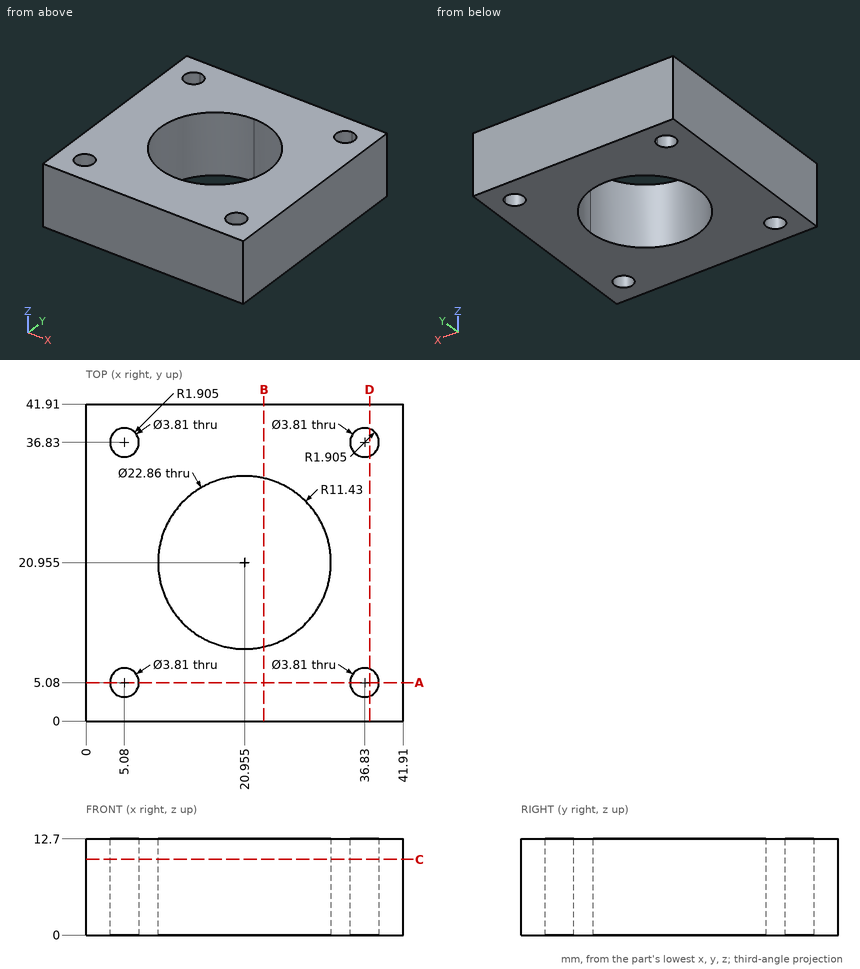
Answer from the drawing. Dimensions are ordinates in mm from the lowest x, y and z of the part. Give positions to 0.01 mm unless a question says otherwise; leave off trailing zeros. Loops run counter-clockwise (first coordinate to the right, second up) from the corner with the lowest first, then second, coordinate; pieces in that order, holes last.
Item 1: Find the intervals of material crossed by line 1 along X through (y, z) = (36.83, 5.5) (3 decimals); line 2 along X through (y, z) = (5.5, 3.5), in increasing order.
Item 2: The part is cut by section A-A (y = 5.08). Write down the section's boundary in (x, z) (3 decimals), and give its area (3 significant figures).
Item 3: The part is cut by section D-D (x = 37.5). Write down the section's boundary in (y, z).
Item 4: The part is cut by section B-B (x = 23.5). Write down the section's boundary in (y, z).
Item 5: The part is cut by section C-C (z = 10). Write down the section's boundary in (x, y) (3 decimals).
Taken from the geometry:
1. line 1: x = 0 to 3.175, 6.985 to 34.925, 38.735 to 41.91
1. line 2: x = 0 to 3.22, 6.94 to 34.97, 38.69 to 41.91
2. outline: (0, 0) - (3.175, 0) - (3.175, 12.7) - (0, 12.7) - close; (6.985, 0) - (34.925, 0) - (34.925, 12.7) - (6.985, 12.7) - close; (38.735, 0) - (41.91, 0) - (41.91, 12.7) - (38.735, 12.7) - close
2. area: 435 mm2
3. outline: (0, 0) - (3.3, 0) - (3.3, 12.7) - (0, 12.7) - close; (6.86, 0) - (35.05, 0) - (35.05, 12.7) - (6.86, 12.7) - close; (38.61, 0) - (41.91, 0) - (41.91, 12.7) - (38.61, 12.7) - close
4. outline: (0, 0) - (9.81, 0) - (9.81, 12.7) - (0, 12.7) - close; (32.1, 0) - (41.91, 0) - (41.91, 12.7) - (32.1, 12.7) - close
5. outline: (0, 0) - (41.91, 0) - (41.91, 41.91) - (0, 41.91) - close; hole circle Ø3.81 at (5.08, 5.08); hole (5.08, 38.735) arc R1.905 ccw (long way) to (6.985, 36.83) arc R1.905 ccw to start; hole (20.955, 32.385) arc R11.43 ccw (long way) to (32.385, 20.955) arc R11.43 ccw to start; hole circle Ø3.81 at (36.83, 5.08); hole (36.83, 38.735) arc R1.905 ccw (long way) to (38.735, 36.83) arc R1.905 ccw to start
